Autodesk Inventor part; units mm, degrees
ref_plane "YZ Plane" through (0, 0, 0) normal (1, 0, 0) x (0, 1, 0)
ref_plane "XZ Plane" through (0, 0, 0) normal (0, 1, 0) x (-1, 0, 0)
ref_plane "XY Plane" through (0, 0, 0) normal (0, 0, 1) x (1, 0, 0)
sketch "Sketch1" plane through (0, 0, 0) normal (0, 1, 0) x (-1, 0, 0)
  line L0 (0, -3.6662) -> (-3.175, -1.8331)
  line L1 (-3.175, -1.8331) -> (-3.175, 1.8331)
  line L2 (-3.175, 1.8331) -> (0, 3.6662)
  line L3 (0, 3.6662) -> (3.175, 1.8331)
  line L4 (3.175, 1.8331) -> (3.175, -1.8331)
  line L5 (3.175, -1.8331) -> (0, -3.6662)
  line L6 (0, 3.6662) -> (0, -3.6662) construction
  point P0 (0, 0)
  point P1 (0, 0)
  dimension "d0" = 6.35
extrude "Extrusion1" add sketch "Sketch1" along normal blind 2.7432
sketch "Sketch2" plane through (0, 2.7432, 0) normal (0, 1, 0) x (1, 0, 0)
  circle A0 centre (0, 0) radius 1.7526
  dimension "d3" = 3.5052
extrude "Extrusion2" cut sketch "Sketch2" against normal blind 2.7432
chamfer "Chamfer1" distance 0.381 angle 45 14 edges at (1.5875, 2.7432, 2.7496) (-1.5875, 2.7432, 2.7496) (-3.175, 2.7432, 0) (-1.5875, 2.7432, -2.7496) (1.5875, 2.7432, -2.7496) (3.175, 2.7432, 0) (-1.7526, 2.7432, 0) (3.175, 0, 0) (1.5875, 0, 2.7496) (-1.5875, 0, 2.7496) (-3.175, 0, 0) (-1.5875, 0, -2.7496) (1.5875, 0, -2.7496) (-1.7526, 0, 0)
thread "Thread1"
properties part number "6-32x0,25 Nut" material "Stainless Steel"
Check sheet for the modelled part. Datum: model origin and axes. Units: mm. Give positions to 0.01 mm unless a question says otherwise; leave off trailing zeros. Write each loop counter-clockwise with the first axis right and the second up, starting at its lowest first coordinate (ties: lowest second). Pieces come first, ordered by that corner, then holes.
Item 1: Gauge pin test, flat end, axial feed: pin 1 (1 mm diameter, centred on x = -1.5, y = 1.5, fed in from -Z). Record the tip position at first contact, or that the pin passes through.
Item 2: Cross-section at B-B (y = 0.9). Enter the section's corners in (x, z) (3 decimals).
Item 3: Cross-section at C-C (z = -2.5). Enter the section's corners in (x, y), and give its area (3 significant figures).
Item 4: Cross-section at A-A (z = 0). Enter the section's corners in (x, y) (3 decimals), and give its area (3 significant figures).
Item 5: Scan lines: L1, parallel to X at y = 1.05, z = 0 (3 decimals); L2, parallel to X at y = 0.85, z = 0.5 (3 decimals); L3, parallel to Z at x = 0.25, y = 1.2. Record each from-to range of solid material in increasing order.
Item 6: Cross-section at D-D (y = 0.2). Enter the section's corners in (x, z), and give its area (3 significant figures).
Item 7: Draft check along Z on faces 1 (the face through (-1.47, 0.19, 2.6)), 2 (the face through (1.67, 1.39, -0.53)), 3 (the face through (-1.61, 1.358, -2.737)). Enter one of: released by +Z, released by -Z, zero draft, split by the parting line, or undercut.
Report:
1. pin 1: stops at z = -3.09
2. outline: (-3.175, -1.833) - (0, -3.666) - (3.175, -1.833) - (3.175, 1.833) - (0, 3.666) - (-3.175, 1.833) - close; hole circle Ø3.505 at (0, 0)
3. outline: (-2.02, 0.38) - (-1.26, 0) - (1.26, 0) - (2.02, 0.38) - (2.02, 2.36) - (1.26, 2.74) - (-1.26, 2.74) - (-2.02, 2.36) - close
3. area: 10.5 mm2
4. outline: (-3.175, 0.381) - (-2.794, 0) - (-2.134, 0) - (-1.753, 0.381) - (-1.753, 2.362) - (-2.134, 2.743) - (-2.794, 2.743) - (-3.175, 2.362) - close; (1.753, 0.381) - (2.134, 0) - (2.794, 0) - (3.175, 0.381) - (3.175, 2.362) - (2.794, 2.743) - (2.134, 2.743) - (1.753, 2.362) - close
4. area: 7.22 mm2
5. L1: x = -3.175 to -1.753, 1.753 to 3.175
5. L2: x = -3.175 to -1.68, 1.68 to 3.175
5. L3: z = -3.52 to -1.73, 1.73 to 3.52
6. outline: (-2.99, -1.73) - (0, -3.46) - (2.99, -1.73) - (2.99, 1.73) - (0, 3.46) - (-2.99, 1.73) - close; hole circle Ø3.87 at (0, 0)
6. area: 19.3 mm2
7. face 1: released by +Z
7. face 2: undercut
7. face 3: released by -Z
